from build123d import *

# Parameters (mm, degrees)
F0_R          = 2
F0_R_2        = 20
F1_DEPTH      = 3
F2_R          = 5
F3_R          = 20
F3_R_2        = 15
F4_DEPTH      = 52
F4_DEPTH_BACK = 8


with BuildPart() as f1:
    # F0 (on Top) → F1 (new body)
    with BuildSketch(Plane.XY):
        with BuildLine():
            ThreePointArc((-13.584878, 19.785123), (-21.92031, 21.92031), (-19.785123, 13.584878))
            ThreePointArc((-19.785123, 13.584878), (-24, 0), (-19.785123, -13.584878))
            ThreePointArc((-19.785123, -13.584878), (-21.92031, -21.92031), (-13.584878, -19.785123))
            ThreePointArc((-13.584878, -19.785123), (0, -24), (13.584878, -19.785123))
            ThreePointArc((13.584878, -19.785123), (21.92031, -21.92031), (19.785123, -13.584878))
            ThreePointArc((19.785123, -13.584878), (24, 0), (19.785123, 13.584878))
            ThreePointArc((19.785123, 13.584878), (21.92031, 21.92031), (13.584878, 19.785123))
            ThreePointArc((13.584878, 19.785123), (0, 24), (-13.584878, 19.785123))
        make_face()
        with Locations((-18.384776, -18.384776)):
            Circle(F0_R, mode=Mode.SUBTRACT)
        with Locations((18.384776, -18.384776)):
            Circle(F0_R, mode=Mode.SUBTRACT)
        with Locations((-18.384776, 18.384776)):
            Circle(F0_R, mode=Mode.SUBTRACT)
        Circle(F0_R_2, mode=Mode.SUBTRACT)
        with Locations((18.384776, 18.384776)):
            Circle(F0_R, mode=Mode.SUBTRACT)
    extrude(amount=F1_DEPTH)

    # F2
    f2_edges = [f1.edges().sort_by_distance(p)[0] for p in [
        (-13.584878, -19.785123, 1.5),
        (19.785123, 13.584878, 1.5),
        (-19.785123, 13.584878, 1.5),
        (-19.785123, -13.584878, 1.5),
        (19.785123, -13.584878, 1.5),
        (-13.584878, 19.785123, 1.5),
        (13.584878, -19.785123, 1.5),
        (13.584878, 19.785123, 1.5),
    ]]
    fillet(f2_edges, radius=F2_R)

    # F3 (on Top) → F4 (join, two sides)
    with BuildSketch(Plane.XY) as f4_sk:
        Circle(F3_R)
        Circle(F3_R_2, mode=Mode.SUBTRACT)
    extrude(amount=F4_DEPTH)
    extrude(f4_sk.sketch, amount=-F4_DEPTH_BACK)


solid = f1.part
Could you check a few things on this model? Use its own coordinates, in mm. A direction names the side the tool comes from. Coordinates: 2 decimals unless noted, no trailing zeros. Loops run counter-clockwise (first coordinate to the right, second up) from the corner with the lowest first, then second, coordinate; pieces in that order, holes last. Notation, with made-up numbers: (25.25, -7) -> (30.25, -7) arc R10 cw to (30.25, 4) -> close; hole circle Ø10 at (28, 16.5). An arc over 180 degrees is marked (long way). Answer in a Markdown table with one row per item.
(1) If I drill on probe 1 along Y at (x, z) = (-18.5, 1); probe 2 along Y at (x, z) = (-3, 35); probe 3 along X at (y, z) = (4.5, 23.5), over which ranges is the centre line in solid material (lowest first)?
Results found:
| item | result |
|---|---|
| probe 1 | y = -23.38 to -20.38, -16.39 to 16.39, 20.38 to 23.38 |
| probe 2 | y = -19.77 to -14.7, 14.7 to 19.77 |
| probe 3 | x = -19.49 to -14.31, 14.31 to 19.49 |
(2) Will these pins go through, and if not, where does the flat tip stop? pin 1 Ø4 at (y, z) = (6, 22) entering from -X; pin 2 Ø5 at (x, z) = (8.5, 2) entering from -Y; pin 3 Ø6.5 at (x, y) = (-18.38, 18.38) entering from -Z.
Results found:
| item | result |
|---|---|
| pin 1 | stops at x = -19.6 |
| pin 2 | stops at y = -23.24 |
| pin 3 | stops at z = 0 |
(3) Imagine slicing it at A-A (y = 0). List the corners of the cut face in (x, z) for me.
Results found:
| item | result |
|---|---|
| outline | (-24, 0) -> (-20, 0) -> (-20, -8) -> (-15, -8) -> (-15, 52) -> (-20, 52) -> (-20, 3) -> (-24, 3) -> close; (15, -8) -> (20, -8) -> (20, 0) -> (24, 0) -> (24, 3) -> (20, 3) -> (20, 52) -> (15, 52) -> close |
(4) Thinking about a two-plate mould opening in Y: for faces 1 (the face through (-4.336, -19.524, -3.944)), 2 (the face through (3, 15, -8)), 3 (the face through (0, -24, 1)), 4 (the face through (21.85, -21.99, 1.48)), which applies, released by +Y, released by -Y, zero draft, split by the parting line, or undercut?
Results found:
| item | result |
|---|---|
| face 1 | split by the parting line |
| face 2 | zero draft |
| face 3 | released by -Y |
| face 4 | undercut |
(5) For faces 5 (the face through (21, 0, 0)), 6 (the face through (-24, 0, 1)), 7 (the face through (-4.336, -19.524, 27.157)), which set-ups out of +Z, -Z, +X, -X, +Y, -Y let a thin tool reach every point of the face, with its end or its side?
Results found:
| item | result |
|---|---|
| face 5 | -Z |
| face 6 | +Z, -Z, -X |
| face 7 | +Z |
(6) Imagine slicing it at C-C (z = 9). List the corners of the cut face in (x, y) for me, plus the area to 3 significant figures.
Results found:
| item | result |
|---|---|
| outline | circle Ø40 at (0, 0); hole circle Ø30 at (0, 0) |
| area | 550 mm^2 |
